Part print with two shaded views. Sizes in mm from the minimum x, y, z corner. A direction names the side the tool comes from. Round coordinates to 2 decimals unless told otherwise and drop trailing zeros. Order: outer loops, then holes, each group sorted by start corner. A loop starts at its lowest first (then second) coordinate and runs counter-clockwise, first axis right, second up. Notation, with made-up numbers: (-34, 83.5) -> (-28, 83.5) arc R14 ccw to (-28, 87.5) -> close; hole circle Ø1 at (49, -18.5). An arc over 180 degrees is marked (long way). Put each result on its own line as item: value. Start each with the question number.
Q1. Flat gauge pin, fed straight in: P1, Ø2, axis at y = 3.5, z = 3.5, coming from the +X side. Where does the tip first touch, or does it go through?
Q2. Pull direction Z, two halves, no side cores. Call the marked faces 3, 4 and 5: released by +Z, released by -Z, zero draft, split by the parting line, or undercut.
Q3. 3-axis set-ups, long thin cutter, end or side, ignore diameter. For the marked faces 1 and 2: which of +Z, -Z, +X, -X, +Y, -Y reach the whole face in a straight line?
Q4. Probe L1, parallel to X at y = 3.1, z = 2.25; L2, parallel to Y at x = 5.5, z = 0.9 (1 decimal); L3, parallel to Y at x = 5.75, z = 2. List the from-to ranges inside material, lowest first.
Q5. Cut at A-A, the plane z = 3. List the corners of the cut face in (x, y), and give its area (3 significant figures).
Q6. Cut at B-B, the plane x = 3. List the corners of the cut face in (y, z).
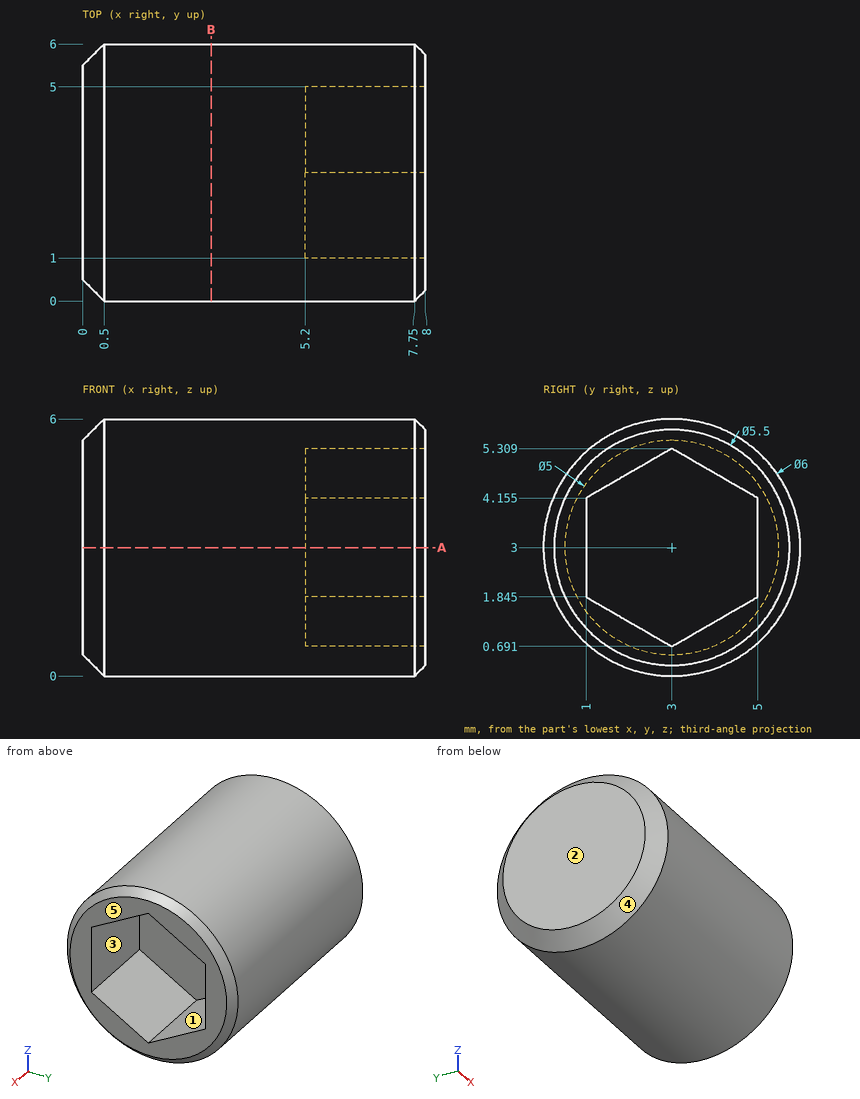
Ans:
1. P1: stops at x = 5.2
2. face 3: undercut
2. face 4: split by the parting line
2. face 5: zero draft
3. face 1: +X
3. face 2: +Z, -Z, -X, +Y, -Y
4. L1: x = 0 to 5.2
4. L2: y = 0.9 to 2.6, 3.4 to 5.1
4. L3: y = 0.17 to 1, 5 to 5.83
5. outline: (0, 0.5) -> (0.5, 0) -> (7.75, 0) -> (8, 0.25) -> (8, 1) -> (5.2, 1) -> (5.2, 5) -> (8, 5) -> (8, 5.75) -> (7.75, 6) -> (0.5, 6) -> (0, 5.5) -> close
5. area: 36.5 mm^2
6. outline: circle Ø6 at (3, 3)
